Input: part model. Units: mm. Frame: model coordinates. Face numbers are marked on the shaded views. Round coordinates to 2 decimals unless told otherwise and drop trailing zeros. Loops run counter-clockwise (first coordinate to the right, second up) from the corner with the lowest first, then second, coordinate; pieces in that order, holes last. Notation, with made-up numbers: (3, 68.25) -> (48, 68.25) arc R22 cw to (48, 85.25) -> close; hole circle Ø6 at (44, 38). An arc over 180 degrees is marked (long way). Answer in a Markdown table with one row per item. Add a question column.
Q1. Mould query, pull axis X, two halves, no side actions, for the marked faces 1, 2, 3 and 4. Classes: pulls with the +X half, pulls with the -X half, needs draft (parallel to the pull), parting line crosses it, or undercut.
Q2. Section A-A, the plane z = -7. Output: boundary loops of the cut face in (x, y).
Q3. Pin query (flat end, axial travel): pin 1 (1.5 mm diameter, centred on x = 7, y = -23, fed in from +Z); pin 2 (1.5 mm diameter, centred on x = 1.5, y = -93.5, fed in from +Z); pin 3 (1 mm diameter, centred on x = 12.5, y = -44, fed in from -Z). Return the tip coordinate at first contact, or that it passes through.
Q4. Section B-B, the plane y = -69.5. Output: boundary loops of the cut face in (x, z), and give its area (3 significant figures).
Q5. Ray query, L1, parallel to X at y = -86, z = -4.75; L2, parallel to Z at x = 13, y = -40.5; L3, parallel to Z at x = 10.25, y = -83. Return the intervals inside material, ascending. Write a range as from..to.
Q6. Section C-C, the plane x = 5.25. Output: boundary loops of the cut face in (y, z).
```python
from build123d import *

# Parameters (mm, degrees)
F1_DEPTH = 100
F2_W     = 3
F2_H     = 1.333333
F2_H_2   = 1.333334
F3_DEPTH = 1


with BuildPart() as f1:
    # F0 (on Front) → F1 (new body)
    with BuildSketch(Plane.XZ):
        Polygon((3, 0), (0, 0), (0, -1), (2, -1), (2, -11), (11.5, -11), (11.5, -1), (13.5, -1), (13.5, 0), (10.5, 0), (10.5, -10), (3, -10), align=None)
    extrude(amount=F1_DEPTH)

    # F2 (on face) → F3 (join)
    with BuildSketch(Plane.XY):
        with Locations((1.5, -0.666666)):
            Rectangle(F2_W, F2_H)
        with Locations((12, -0.666666)):
            Rectangle(F2_W, F2_H)
        with Locations((1.5, -13)):
            Rectangle(F2_W, F2_H_2)
        with Locations((12, -13)):
            Rectangle(F2_W, F2_H_2)
        with Locations((1.5, -25.333334)):
            Rectangle(F2_W, F2_H)
        with Locations((12, -25.333334)):
            Rectangle(F2_W, F2_H)
        with Locations((1.5, -37.666666)):
            Rectangle(F2_W, F2_H)
        with Locations((12, -37.666666)):
            Rectangle(F2_W, F2_H)
        with Locations((1.5, -50)):
            Rectangle(F2_W, F2_H_2)
        with Locations((12, -50)):
            Rectangle(F2_W, F2_H_2)
        with Locations((1.5, -62.333333)):
            Rectangle(F2_W, F2_H)
        with Locations((12, -62.333333)):
            Rectangle(F2_W, F2_H)
        with Locations((1.5, -74.666666)):
            Rectangle(F2_W, F2_H)
        with Locations((12, -74.666666)):
            Rectangle(F2_W, F2_H)
        with Locations((1.5, -87)):
            Rectangle(F2_W, F2_H_2)
        with Locations((12, -87)):
            Rectangle(F2_W, F2_H_2)
        with Locations((1.5, -99.333333)):
            Rectangle(F2_W, F2_H)
        with Locations((12, -99.333333)):
            Rectangle(F2_W, F2_H)
    extrude(amount=F3_DEPTH)


solid = f1.part
```
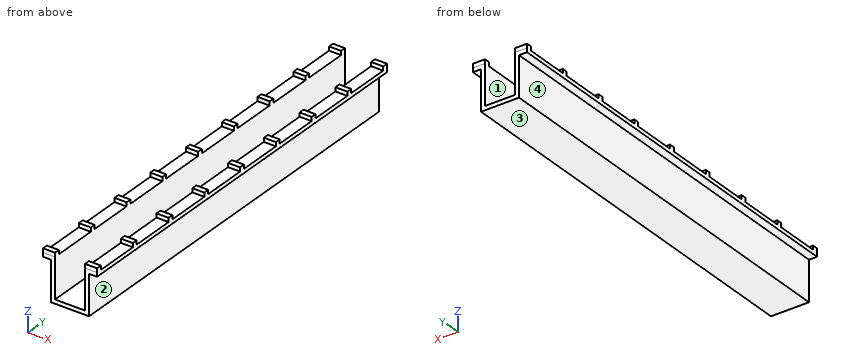
Answer block:
| question | item | result |
|---|---|---|
| 1 | face 1 | undercut |
| 1 | face 2 | pulls with the +X half |
| 1 | face 3 | needs draft |
| 1 | face 4 | pulls with the -X half |
| 2 | outline | (2, -100) -> (3, -100) -> (3, 0) -> (2, 0) -> close; (10.5, -100) -> (11.5, -100) -> (11.5, 0) -> (10.5, 0) -> close |
| 3 | pin 1 | z = -10 |
| 3 | pin 2 | z = 0 |
| 3 | pin 3 | z = -1 |
| 4 | outline | (0, -1) -> (2, -1) -> (2, -11) -> (11.5, -11) -> (11.5, -1) -> (13.5, -1) -> (13.5, 0) -> (10.5, 0) -> (10.5, -10) -> (3, -10) -> (3, 0) -> (0, 0) -> close |
| 4 | area | 33.5 mm^2 |
| 5 | L1 | 2..3, 10.5..11.5 |
| 5 | L2 | -1..0 |
| 5 | L3 | -11..-10 |
| 6 | outline | (-100, -11) -> (0, -11) -> (0, -10) -> (-100, -10) -> close |
